Input: part model. Units: mm. Frame: model coordinates. Give positions to 0.01 mm unless a question says otherwise; leave off trailing zeros. Order: outer loops, then holes, each group sorted by start corner. A loop starts at its lowest first (then second) coordinate and runs counter-clockwise, first axis right, second up. Notation, with made-up numbers: (58, -19.5) -> (68, -19.5) arc R26 cw to (68, 11.5) -> close; hole circle Ø7 at (48.5, -30.75). An arc over 180 degrees is marked (long way). Use a Markdown table: item, result. Add a question column.
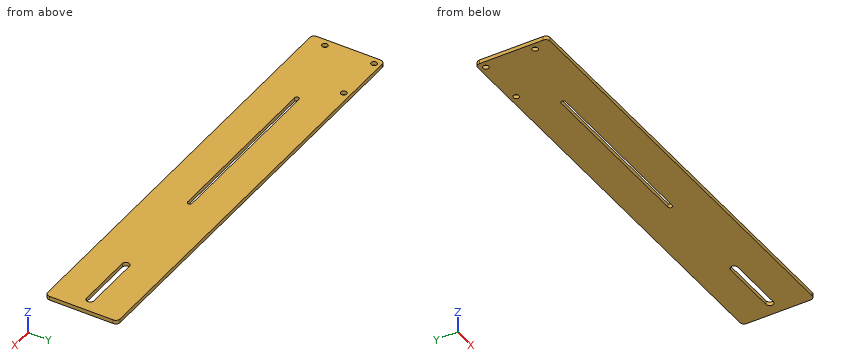
from build123d import *

# Parameters (mm, degrees)
SKETCH_1_R      = 2
EXTRUDE_1_DEPTH = 2.7


with BuildPart() as part:
    # 草图1 → 凸台-拉伸1 (new body)
    with BuildSketch(Plane.XY):
        with BuildLine():
            Line((0, 22), (0, -22))
            ThreePointArc((0, -22), (0.878679656, -24.121320344), (3, -25))
            Line((3, -25), (297, -25))
            ThreePointArc((297, -25), (299.121320344, -24.121320344), (300, -22))
            Line((300, -22), (300, 22))
            ThreePointArc((300, 22), (299.121320344, 24.121320344), (297, 25))
            Line((297, 25), (3, 25))
            ThreePointArc((3, 25), (0.878679656, 24.121320344), (0, 22))
        make_face()
        with Locations(Location((5, 20.65, 0), (0, 0, 180))):
            Circle(SKETCH_1_R, mode=Mode.SUBTRACT)
        with Locations(Location((39, 20.65, 0), (0, 0, 180))):
            Circle(SKETCH_1_R, mode=Mode.SUBTRACT)
        with Locations(Location((5, -13.35, 0), (0, 0, 180))):
            Circle(SKETCH_1_R, mode=Mode.SUBTRACT)
        with BuildLine():
            Line((250, 2.5), (290, 2.5))
            ThreePointArc((290, 2.5), (292.5, 0), (290, -2.5))
            Line((290, -2.5), (250, -2.5))
            ThreePointArc((250, -2.5), (247.5, 0), (250, 2.5))
        make_face(mode=Mode.SUBTRACT)
        with BuildLine():
            Line((58.219392868, 1.5), (178.219392868, 1.5))
            ThreePointArc((178.219392868, 1.5), (179.719392868, 0), (178.219392868, -1.5))
            Line((178.219392868, -1.5), (58.219392868, -1.5))
            ThreePointArc((58.219392868, -1.5), (56.719392868, 0), (58.219392868, 1.5))
        make_face(mode=Mode.SUBTRACT)
    extrude(amount=EXTRUDE_1_DEPTH)


solid = part.part
Q1. Section query B-B (z = 1.6). Return loops of the section in (x, y).
Q2. Section query A-A (x = 61.5). Return loops of the section in (y, z).
Q3. Ray query, line 1 (X direction, y = 20.5, z = 1.15); line 2 (X direction, y = -13.35, z = 1.25); line 3 (Y direction, x = 75, z = 1.05). Return the intervals inside material, ascending.
Solution:
| question | item | result |
|---|---|---|
| 1 | outline | (0, -22) arc R3 ccw to (3, -25) -> (297, -25) arc R3 ccw to (300, -22) -> (300, 22) arc R3 ccw to (297, 25) -> (3, 25) arc R3 ccw to (0, 22) -> close; hole circle Ø4 at (5, -13.35); hole circle Ø4 at (5, 20.65); hole circle Ø4 at (39, 20.65); hole (58.22, -1.5) -> (178.22, -1.5) arc R1.5 ccw to (178.22, 1.5) -> (58.22, 1.5) arc R1.5 ccw to start; hole (250, -2.5) -> (290, -2.5) arc R2.5 ccw to (290, 2.5) -> (250, 2.5) arc R2.5 ccw to start |
| 2 | outline | (-25, 0) -> (-1.5, 0) -> (-1.5, 2.7) -> (-25, 2.7) -> close; (1.5, 0) -> (25, 0) -> (25, 2.7) -> (1.5, 2.7) -> close |
| 3 | line 1 | x = 0 to 3.01, 6.99 to 37.01, 40.99 to 300 |
| 3 | line 2 | x = 0 to 3, 7 to 300 |
| 3 | line 3 | y = -25 to -1.5, 1.5 to 25 |
